Source: CAD feature listing. Evaluate the final solid. Frame: model axes, mm. A direction names the side the tool comes from. Round coordinates to 2 decimals unless told otherwise and drop trailing zeros. Order: outer loops, then holes, each group sorted by start corner. A loop starts at its lowest first (then second) coordinate and runs counter-clockwise, first axis right, second up. Notation, with made-up numbers: M 8.5,85.25 L 46.5,85.25 A3 ccw 46.5,89.25 Z; hole C 36,88 d3. An arc over 180 degrees is marked long. Use CSV: the item, a comma, the result in double quotes. Start each with the question number.
```python
from build123d import *

# Parameters (mm, degrees)
F0_W     = 31.75
F0_H     = 50.8
F1_DEPTH = 6.604
F2_SIZE2 = 31.433603
F2_SIZE  = 12.7
F4_DEPTH = 38.1


with BuildPart() as f1:
    # F0 (on Right) → F1 (new body)
    with BuildSketch(Plane.YZ):
        with Locations((-15.875, -3.497973)):
            Rectangle(F0_W, F0_H)
    extrude(amount=F1_DEPTH)

    # F2
    f2_edges = [f1.edges().sort_by_distance(p)[0] for p in [
        (3.302, -31.75, -28.897973),
    ]]
    chamfer(f2_edges, length=F2_SIZE, length2=F2_SIZE2)

    # F3 (on face) → F4 (cut)
    with BuildSketch(Plane.XY.offset(21.902027)):
        Polygon((0.762, -30.48), (3.302, -30.48), (5.842, -30.48), (5.842, -1.27), (3.302, -1.27), (0.762, -1.27), align=None)
    extrude(amount=-F4_DEPTH, mode=Mode.SUBTRACT)


solid = f1.part
```
(1) Section D-D on z = -23. Return loops of the section in (x, y).
(2) Section A-A on z = -14. Return loops of the section in (x, y).
(3) Section C-C on y = -8. Return loops of the section in (x, z).
(4) Reachability of faces 1 (the face through (3, -30.48, 3)), 2 (the face through (0, -16, 3)) from +Z, -Z, +X, -X, +Y, -Y: full face, straight path, thin tool, end or side. Return the list, or none.
(5) Line query: line 1 along X through (y, z) = (-13, 14); line 2 along Y through (x, z) = (4.75, -7). Output: solid intervals per line, ascending.
(6) Contact query for flat-ended pins moving along their axis: P1, Ø1.5, axis at x = 4.5, z = -4, coming from the +Y side; P2, Ø2.5, axis at x = 4, y = -14, coming from the +Z side. Output: stop coordinate, or through.
(7) Section B-B on x = 2.25. Return loops of the section in (y, z), plus the area to 3 significant figures.
Results below:
1,outline,"M 0,-14.91 L 6.6,-14.91 L 6.6,0 L 0,0 Z"
2,outline,"M 0,-31.75 L 6.6,-31.75 L 6.6,0 L 0,0 Z; hole M 0.76,-30.48 L 5.84,-30.48 L 5.84,-1.27 L 0.76,-1.27 Z"
3,outline,"M 0,-25.79 L 6.6,-25.79 L 6.6,21.9 L 5.84,21.9 L 5.84,-16.2 L 0.76,-16.2 L 0.76,21.9 L 0,21.9 Z"
4,face 1,"+Z"
4,face 2,"+Z, -Z, -X, +Y, -Y"
5,line 1,"x = 0 to 0.76, 5.84 to 6.6"
5,line 2,"y = -31.75 to -30.48, -1.27 to 0"
6,P1,"stops at y = 0"
6,P2,"stops at z = -16.2"
7,outline,"M -31.75,-16.2 L -0.32,-28.9 L 0,-28.9 L 0,21.9 L -1.27,21.9 L -1.27,-16.2 L -30.48,-16.2 L -30.48,21.9 L -31.75,21.9 Z"
7,area,"300 mm2"
